Could you check a few things on this model? Use its own coordinates, in mm. A direction names the side the tool comes from. Round coordinates to 2 decimals unless told otherwise and drop trailing zeros. Loops run counter-clockwise (first coordinate to the right, second up) from the corner with the lowest first, then second, coordinate; pieces in that order, holes last. Notation, with made-up numbers: (-20.5, -31.75) - (9.5, -31.75) arc R16 ccw to (9.5, -16.75) - close; hole circle Ø1 at (-28.75, 84.25). An arc over 180 degrees is marked (long way). Answer as CSV lines item,"result". Start each with the question number.
1) Please list where these lines run through material, in increasing order: line 1 along X through (y, z) = (30.5, -50.5); line 2 along Y through (x, z) = (11.1, -46.5); line 3 along Z through (x, y) = (45.5, 8).
2) Suppose I cut it at D-D, the plane y = 24. Write out the boundary of the cut face in (x, z).
3) We'd pull the mould along Z, two halves only. Please class faces 4 (the face through (27.273, 45.542, -3.716)), 5 (the face through (31, 16, -10)), 6 (the face through (62.2, 43, -8.5)), 7 (the face through (2.03, 22.18, -7.39)): pulls with the +Z half, pulls with the -Z half, needs draft (parallel to the pull), parting line crosses it, or undercut.
4) Suppose I cut it at B-B, the plane y = 15.65. Count the separate pieces of the cut face and the enclosed holes in it, then the cut area to 3 significant figures.
5) I'm going to push flat-ended pins straight in: pin 1 Ø5 at (x, z) = (46, -60.5) entering from -Y; pin 2 Ø6 at (x, z) = (66.5, -13) entering from +Y; pin 3 Ø3 at (x, z) = (49, -64) entering from +Y; pin 4 Ø4 at (y, z) = (35.5, -7.5) entering from -X. Where does each tip first touch, or does it pass through?
6) Suppose I cut it at A-A, the plane z = -37. Write out the boundary of the cut face in (x, y).
7) Suppose I cut it at C-C, the plane x = 47. Write out the boundary of the cut face in (y, z).
8) Which directions (+Z, -Z, +X, -X, +Y, -Y) give clear straight access to the entire face, cutting with the end or side of a thin tool? Please do faces 1 (the face through (31, 16, -60)), 2 (the face through (4.93, 40.34, -25.34)), 3 (the face through (22.6, 43, -8.5)).
```python
from build123d import *
from OCP.BRepFilletAPI import BRepFilletAPI_MakeChamfer

# Parameters (mm, degrees)
SKETCH1_W           = 90
SKETCH1_H           = 70
BOSS_EXTRUDE1_DEPTH = 46
SKETCH2_W           = 53
SKETCH2_H           = 50
CUT_EXTRUDE1_DEPTH  = 123.947143114
SKETCH3_R           = 3
CUT_EXTRUDE2_DEPTH  = 123.947143114
SKETCH4_W           = 23
SKETCH4_H           = 36
CUT_EXTRUDE3_DEPTH  = 123.947143114
CHAMFER1_SIZE       = 10
CHAMFER1_SIZE2      = 4
CHAMFER2_SIZE       = 4
CHAMFER2_SIZE2      = 10
CHAMFER3_SIZE       = 3
CHAMFER3_SIZE_2     = 6
CHAMFER4_SIZE       = 4
CHAMFER4_SIZE2      = 15
CHAMFER5_SIZE       = 15
CHAMFER5_SIZE2      = 4
CHAMFER6_SIZE       = 1
CHAMFER6_SIZE2      = 1.795054936
CHAMFER7_SIZE       = 0.5
SKETCH5_R           = 2.5
CUT_EXTRUDE4_DEPTH  = 10
SKETCH7_R           = 4
CUT_EXTRUDE5_DEPTH  = 5


with BuildPart() as part:
    # Sketch1 → Boss-Extrude1 (new body)
    with BuildSketch(Plane(origin=(0, 0, 0), x_dir=(1, 0, 0), z_dir=(0, 1, 0))):
        with Locations((45, 35)):
            Rectangle(SKETCH1_W, SKETCH1_H)
    extrude(amount=BOSS_EXTRUDE1_DEPTH)

    # Sketch2 → Cut-Extrude1 (cut, through all)
    with BuildSketch(Plane(origin=(0, 46, 0), x_dir=(1, 0, 0), z_dir=(0, 1, 0))):
        with Locations((41.5, 35)):
            Rectangle(SKETCH2_W, SKETCH2_H)
    extrude(amount=-CUT_EXTRUDE1_DEPTH, mode=Mode.SUBTRACT)

    # Sketch3 → Cut-Extrude2 (cut, through all)
    with BuildSketch(Plane(origin=(0, 46, 0), x_dir=(1, 0, 0), z_dir=(0, 1, 0))):
        with Locations((15, 60)):
            Circle(SKETCH3_R)
        with Locations((68, 60)):
            Circle(SKETCH3_R)
        with Locations((68, 10)):
            Circle(SKETCH3_R)
        with Locations((15, 10)):
            Circle(SKETCH3_R)
    extrude(amount=-CUT_EXTRUDE2_DEPTH, mode=Mode.SUBTRACT)

    # Sketch4 → Cut-Extrude3 (cut, through all)
    with BuildSketch(Plane.XY):
        with Locations((43.5, 28)):
            Rectangle(SKETCH4_W, SKETCH4_H)
    extrude(amount=-CUT_EXTRUDE3_DEPTH, mode=Mode.SUBTRACT)

    # Chamfer1: one chamfer whose edges measure the first distance from different faces: ONE call of the kernel's chamfer builder (chamfer() names one face for all edges)
    chamfer1_edges_1 = [part.edges().sort_by_distance(p)[0] for p in [
        (55, 46, -65),
    ]]
    chamfer1_side_1 = [part.faces().sort_by_distance(p)[0] for p in [
        (55, 28, -65),
    ]]
    chamfer1_edges_2 = [part.edges().sort_by_distance(p)[0] for p in [
        (55, 46, -5),
    ]]
    chamfer1_side_2 = [part.faces().sort_by_distance(p)[0] for p in [
        (55, 28, -5),
    ]]
    chamfer1 = BRepFilletAPI_MakeChamfer(part.part.solid().wrapped)
    for e in chamfer1_edges_1:
        chamfer1.Add(CHAMFER1_SIZE, CHAMFER1_SIZE2, e.wrapped, chamfer1_side_1[0].wrapped)  # the first distance lies on this face
    for e in chamfer1_edges_2:
        chamfer1.Add(CHAMFER1_SIZE, CHAMFER1_SIZE2, e.wrapped, chamfer1_side_2[0].wrapped)  # the first distance lies on this face
    add(Compound.cast(chamfer1.Shape()), mode=Mode.REPLACE)

    # Chamfer2
    chamfer2_edges = [part.edges().sort_by_distance(p)[0] for p in [
        (32, 46, -65),
        (32, 46, -5),
    ]]
    chamfer2_side = [part.faces().sort_by_distance(p)[0] for p in [
        (11.31415673, 46, -35),
    ]]
    chamfer(chamfer2_edges, length=CHAMFER2_SIZE, length2=CHAMFER2_SIZE2, reference=chamfer2_side[0])

    # Chamfer3
    chamfer3_edges_1 = [part.edges().sort_by_distance(p)[0] for p in [
        (62, 46, -10),
    ]]
    chamfer3_side_1 = [part.faces().sort_by_distance(p)[0] for p in [
        (62, 46, -9.94),
    ]]
    chamfer3_edges_2 = [part.edges().sort_by_distance(p)[0] for p in [
        (68, 46, -35),
    ]]
    chamfer3_side_2 = [part.faces().sort_by_distance(p)[0] for p in [
        (68.06, 46, -35),
    ]]
    chamfer3_edges_3 = [part.edges().sort_by_distance(p)[0] for p in [
        (62, 46, -60),
    ]]
    chamfer3_side_3 = [part.faces().sort_by_distance(p)[0] for p in [
        (62, 46, -60.06),
    ]]
    chamfer3_edges_4 = [part.edges().sort_by_distance(p)[0] for p in [
        (23, 46, -60),
    ]]
    chamfer3_side_4 = [part.faces().sort_by_distance(p)[0] for p in [
        (23, 46, -60.06),
    ]]
    chamfer3_edges_5 = [part.edges().sort_by_distance(p)[0] for p in [
        (23, 46, -10),
    ]]
    chamfer3_side_5 = [part.faces().sort_by_distance(p)[0] for p in [
        (23, 46, -9.94),
    ]]
    chamfer3_edges_6 = [part.edges().sort_by_distance(p)[0] for p in [
        (15, 46, -35),
    ]]
    chamfer3_side_6 = [part.faces().sort_by_distance(p)[0] for p in [
        (14.94, 46, -35),
    ]]
    chamfer3 = BRepFilletAPI_MakeChamfer(part.part.solid().wrapped)
    for e in chamfer3_edges_1:
        chamfer3.Add(CHAMFER3_SIZE - 0.0001, CHAMFER3_SIZE_2 - 0.0001, e.wrapped, chamfer3_side_1[0].wrapped)
    for e in chamfer3_edges_2:
        chamfer3.Add(CHAMFER3_SIZE - 0.0001, CHAMFER3_SIZE_2 - 0.0001, e.wrapped, chamfer3_side_2[0].wrapped)
    for e in chamfer3_edges_3:
        chamfer3.Add(CHAMFER3_SIZE - 0.0001, CHAMFER3_SIZE_2 - 0.0001, e.wrapped, chamfer3_side_3[0].wrapped)
    for e in chamfer3_edges_4:
        chamfer3.Add(CHAMFER3_SIZE - 0.0001, CHAMFER3_SIZE_2 - 0.0001, e.wrapped, chamfer3_side_4[0].wrapped)
    for e in chamfer3_edges_5:
        chamfer3.Add(CHAMFER3_SIZE - 0.0001, CHAMFER3_SIZE_2 - 0.0001, e.wrapped, chamfer3_side_5[0].wrapped)
    for e in chamfer3_edges_6:
        chamfer3.Add(CHAMFER3_SIZE - 0.0001, CHAMFER3_SIZE_2 - 0.0001, e.wrapped, chamfer3_side_6[0].wrapped)
    add(Compound.cast(chamfer3.Shape()), mode=Mode.REPLACE)  # a hair under: the kernel refuses the full size

    # Chamfer4
    chamfer4_edges = [part.edges().sort_by_distance(p)[0] for p in [
        (0, 23, -70),
    ]]
    chamfer4_side = [part.faces().sort_by_distance(p)[0] for p in [
        (30.989257699, 23, -70),
    ]]
    chamfer(chamfer4_edges, length=CHAMFER4_SIZE, length2=CHAMFER4_SIZE2, reference=chamfer4_side[0])

    # Chamfer5
    chamfer5_edges = [part.edges().sort_by_distance(p)[0] for p in [
        (0, 23, 0),
    ]]
    chamfer5_side = [part.faces().sort_by_distance(p)[0] for p in [
        (0, 23, -27.5),
    ]]
    chamfer(chamfer5_edges, length=CHAMFER5_SIZE, length2=CHAMFER5_SIZE2, reference=chamfer5_side[0])

    # Chamfer6: one chamfer whose edges measure the first distance from different faces: ONE call of the kernel's chamfer builder (chamfer() names one face for all edges)
    chamfer6_edges_1 = [part.edges().sort_by_distance(p)[0] for p in [
        (16, 46, -70),
        (0, 46, -35),
        (2, 46, -62.5),
        (16, 46, 0),
        (2, 46, -7.5),
    ]]
    chamfer6_edges_2 = [part.edges().sort_by_distance(p)[0] for p in [
        (28, 46, -3.50005),
    ]]
    chamfer6_side_2 = [part.faces().sort_by_distance(p)[0] for p in [
        (30.118676116, 40.703309709, -4.604414044),
    ]]
    chamfer6_edges_3 = [part.edges().sort_by_distance(p)[0] for p in [
        (28, 46, -66.49995),
    ]]
    chamfer6_side_3 = [part.faces().sort_by_distance(p)[0] for p in [
        (30.118676116, 40.703309709, -65.395585956),
    ]]
    chamfer6 = BRepFilletAPI_MakeChamfer(part.part.solid().wrapped)
    for e in chamfer6_edges_1:
        chamfer6.Add(CHAMFER6_SIZE, e.wrapped)
    for e in chamfer6_edges_2:
        chamfer6.Add(CHAMFER6_SIZE, CHAMFER6_SIZE2, e.wrapped, chamfer6_side_2[0].wrapped)  # the first distance lies on this face
    for e in chamfer6_edges_3:
        chamfer6.Add(CHAMFER6_SIZE, CHAMFER6_SIZE2, e.wrapped, chamfer6_side_3[0].wrapped)  # the first distance lies on this face
    add(Compound.cast(chamfer6.Shape()), mode=Mode.REPLACE)

    # Chamfer7
    chamfer7_edges = [part.edges().sort_by_distance(p)[0] for p in [
        (74.5, 46, 0),
        (90, 46, -35),
        (74.5, 46, -70),
    ]]
    chamfer(chamfer7_edges, length=CHAMFER7_SIZE)

    # Sketch5 → Cut-Extrude4 (cut)
    with BuildSketch(Plane.ZY):
        with Locations((-23.5, 38.65)):
            Circle(SKETCH5_R)
        with Locations((-46.5, 15.65)):
            Circle(SKETCH5_R)
    extrude(amount=-CUT_EXTRUDE4_DEPTH, mode=Mode.SUBTRACT)

    # Sketch7 → Cut-Extrude5 (cut)
    with BuildSketch(Plane(origin=(15, 0, 0), x_dir=(0, 0, -1), z_dir=(1, 0, 0))):
        with Locations((23.5, 38.65)):
            Circle(SKETCH7_R)
        with Locations((46.5, 15.65)):
            Circle(SKETCH7_R)
    extrude(amount=-CUT_EXTRUDE5_DEPTH, mode=Mode.SUBTRACT)


solid = part.part
```
Filled sheet:
1,line 1,"0 to 15, 68 to 90"
1,line 2,"0 to 11.65, 19.65 to 46"
1,line 3,"-70 to -60, -10 to 0"
2,outline,"(0, -55) - (4, -70) - (32, -70) - (32, -60) - (18, -60) arc R3 cw (long way) to (15, -57) - (15, -13) arc R3 cw (long way) to (18, -10) - (32, -10) - (32, 0) - (4, 0) - (0, -15) - close; (55, -70) - (90, -70) - (90, 0) - (55, 0) - (55, -10) - (65, -10) arc R3 cw (long way) to (68, -13) - (68, -57) arc R3 cw (long way) to (65, -60) - (55, -60) - close"
3,face 4,"needs draft"
3,face 5,"undercut"
3,face 6,"undercut"
3,face 7,"pulls with the +Z half"
4,separate pieces,"3"
4,enclosed holes,"0"
4,area,"2,960 mm²"
5,pin 1,"y = 0"
5,pin 2,"y = 43"
5,pin 3,"y = 10"
5,pin 4,"x = 1.47"
6,outline,"(0, 0) - (15, 0) - (15, 40) - (12, 46) - (1, 46) - (0, 45) - close; (68, 0) - (90, 0) - (90, 45.5) - (89.5, 46) - (71, 46) - (68, 40) - close"
7,outline,"(0, -70) - (10, -70) - (10, -60) - (0, -60) - close; (0, -10) - (10, -10) - (10, 0) - (0, 0) - close"
8,face 1,"+Y, -Y"
8,face 2,"-X"
8,face 3,"+Y"
